Autodesk Inventor part; units mm, degrees
ref_plane "YZ Plane" through (0, 0, 0) normal (1, 0, 0) x (0, 1, 0)
ref_plane "XZ Plane" through (0, 0, 0) normal (0, 1, 0) x (-1, 0, 0)
ref_plane "XY Plane" through (0, 0, 0) normal (0, 0, 1) x (1, 0, 0)
sketch "Sketch6" plane through (0, 0, 0) normal (0, 0, 1) x (1, 0, 0)
  line L0 (18, 18) -> (-18, 18)
  line L1 (-18, 18) -> (-18, -18)
  line L2 (-18, -18) -> (18, -18)
  line L3 (18, -18) -> (18, 18)
  line L4 (18, 18) -> (-18, -18) construction
  circle A0 centre (0, -34) radius 5.05
  circle A1 centre (35, 20) radius 5.05
  circle A2 centre (-35, 20) radius 5.05
  line L5 (35, 20) -> (-35, 20) construction
  line L6 (-35, 20) -> (0, -34) construction
  line L7 (0, -34) -> (35, 20) construction
  line L8 (0, 18) -> (0, -18) construction
  line L9 (-47.5046, 28) -> (47.5046, 28)
  line L10 (-18, 18) -> (23.6569, -23.6569) construction
  line L11 (18, 18) -> (-23.6569, -23.6569) construction
  line L12 (47.5046, 28) -> (23.6569, -23.6569)
  line L13 (23.6569, -23.6569) -> (0, -44.709)
  line L14 (0, -44.709) -> (-23.6569, -23.6569)
  line L15 (-47.5046, 28) -> (-23.6569, -23.6569)
  line L16 (-35, 20) -> (-42.2633, 16.6468) construction
  line L17 (0, -34) -> (-5.3183, -39.9763) construction
  point P0 (0, 0)
  point P1 (0, 0)
  point P2 (60, 0)
  point P3 (0, 28)
  point P4 (0, 0)
  dimension "d30" = 36
  dimension "d31" = 36
  dimension "d33" = 10.1
  dimension "d37" = 64.3506
  dimension "d52" = 70
  dimension "d53" = 8
  dimension "d54" = 20
  dimension "d57" = 8
  dimension "d59" = 8
  dimension "d60" = 95.0092
  dimension "d61" = 54
  dimension "d62" = 8
  dimension "d63" = 8
  dimension "d64" = 10
extrude "Plate3" add sketch "Sketch6" along normal blind 3
fillet "Corner Round2" radius 6 5 edges at (-47.5046, 28, 1.5) (47.5046, 28, 1.5) (0, -44.709, 1.5) (-23.6569, -23.6569, 1.5) (23.6569, -23.6569, 1.5)
equation "\"d41\" = Thickness"
equation "\"BendReliefWidth\" = Thickness"
equation "\"BendReliefDepth\" = 0.5 * Thickness"
equation "\"CornerReliefSize\" = 4 * Thickness"
equation "\"MinimumRemnant\" = 2 * Thickness"
equation "\"TransitionRadius\" = BendRadius"
equation "\"JacobiRadiusSize\" = BendRadius"
equation "\"GapSize\" = Thickness"
properties part number "DSB-507 beam flange" material "Stainless Steel"
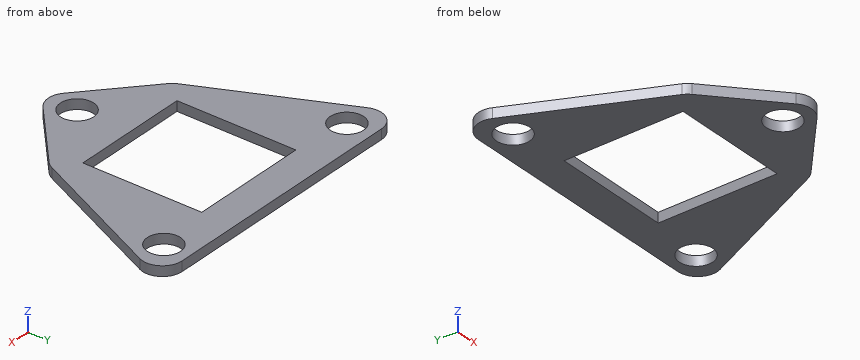
Input: part model. Units: mm. Frame: model coordinates. Coordinates: 2 decimals unless noted, no trailing zeros. Loops run counter-clockwise (first coordinate to the right, second up) from the corner with the lowest first, then second, coordinate; pieces in that order, holes last.
Q1. Section C-C, the plane y = 16. Return the cut outline in (x, z), and give its area (3 significant figures).
Results are:
outline: (-41.96, 0) - (-38.08, 0) - (-38.08, 3) - (-41.96, 3) - close; (-31.92, 0) - (-18, 0) - (-18, 3) - (-31.92, 3) - close; (18, 0) - (31.92, 0) - (31.92, 3) - (18, 3) - close; (38.08, 0) - (41.96, 0) - (41.96, 3) - (38.08, 3) - close
area: 107 mm2
Q2. Section A-A, the plane x = 0. Return the cut outline in (y, z).
Results are:
outline: (-42.68, 0) - (-39.05, 0) - (-39.05, 3) - (-42.68, 3) - close; (-28.95, 0) - (-18, 0) - (-18, 3) - (-28.95, 3) - close; (18, 0) - (28, 0) - (28, 3) - (18, 3) - close
Q3. Section B-B, the plane z = 2.05. Return the cut outline in (x, y).
Results are:
outline: (-43.57, 19.49) - (-24.18, -22.52) arc R6 ccw to (-22.72, -24.49) - (-3.99, -41.16) arc R6 ccw to (3.99, -41.16) - (22.72, -24.49) arc R6 ccw to (24.18, -22.52) - (43.57, 19.49) arc R6 ccw to (38.13, 28) - (-38.13, 28) arc R6 ccw to start; hole circle Ø10.1 at (-35, 20); hole (-18, -18) - (18, -18) - (18, 18) - (-18, 18) - close; hole circle Ø10.1 at (0, -34); hole circle Ø10.1 at (35, 20)
Q4. Contact query for flat-ended pins moving along their axis: pin 1 (8 mm diameter, centred on x = 35, y = 20, fed in from -Z); pin 2 (12 mm diameter, centred on x = 8.5, y = -34, fed in from -Z); pin 3 (0.9 mm diameter, centred on x = 2, z = 2, fed in from -Y). Output: stop coordinate, or through.
Results are:
pin 1: passes through
pin 2: stops at z = 0
pin 3: stops at y = -42.47
Q5. Line query: line 1 along Y through (x, z) = (0, 1.05); line 2 along Y through (x, z) = (-11, 0.35); line 3 along Y through (x, z) = (1.5, 2.1). Output: solid intervals per line, ascending.
Results are:
line 1: y = -42.68 to -39.05, -28.95 to -18, 18 to 28
line 2: y = -34.92 to -18, 18 to 28
line 3: y = -42.49 to -38.82, -29.18 to -18, 18 to 28
Q6. Section D-D, the plane x = 37. Return the cut outline in (y, z), and give its area (3 significant figures).
Results are:
outline: (5.25, 0) - (15.36, 0) - (15.36, 3) - (5.25, 3) - close; (24.64, 0) - (28, 0) - (28, 3) - (24.64, 3) - close
area: 40.4 mm2
